from build123d import *

# Parameters (mm, degrees)
BOSS_EXTRUDE1_DEPTH = 6.35
SKETCH3_R           = 12.7
CUT_EXTRUDE1_DEPTH  = 3.175
SKETCH5_R           = 12.7
CUT_EXTRUDE2_DEPTH  = 3.175
SKETCH6_R           = 3.175
BOSS_EXTRUDE2_DEPTH = 25.4
FILLET1_R           = 2.54


with BuildPart() as part:
    # Sketch2 → Boss-Extrude1 (new body)
    with BuildSketch(Plane(origin=(0, 0, 0), x_dir=(1, 0, 0), z_dir=(0, 1, 0))):
        with BuildLine():
            ThreePointArc((0, -6.090706035), (29.21, 0), (0, 6.090706035))
            ThreePointArc((0, 6.090706035), (-29.21, 0), (0, -6.090706035))
        make_face()
    extrude(amount=BOSS_EXTRUDE1_DEPTH)

    # Sketch3 → Cut-Extrude1 (cut)
    with BuildSketch(Plane(origin=(0, 6.35, 0), x_dir=(1, 0, 0), z_dir=(0, 1, 0))):
        with Locations(Location((-13.959659088, 0, 0), (0, 0, 270))):
            Circle(SKETCH3_R)
    extrude(amount=-CUT_EXTRUDE1_DEPTH, mode=Mode.SUBTRACT)

    # Sketch5 → Cut-Extrude2 (cut)
    with BuildSketch(Plane(origin=(0, 6.35, 0), x_dir=(1, 0, 0), z_dir=(0, 1, 0))):
        with Locations(Location((14.045562682, 0, 0), (0, 0, 270))):
            Circle(SKETCH5_R)
    extrude(amount=-CUT_EXTRUDE2_DEPTH, mode=Mode.SUBTRACT)

    # Sketch6 → Boss-Extrude2 (add)
    with BuildSketch(Plane(origin=(0, 0, 0), x_dir=(-1, 0, 0), z_dir=(0, -1, 0))):
        with Locations(Location((0, 0, 0), (0, 0, 270))):
            Circle(SKETCH6_R)
    extrude(amount=BOSS_EXTRUDE2_DEPTH)

    # Fillet1
    fillet1_edges = [part.edges().sort_by_distance(p)[0] for p in [
        (0, 0, -3.175),
        (0, 3.175, -6.090706035),
        (0, 3.175, 6.090706035),
    ]]
    fillet(fillet1_edges, radius=FILLET1_R)


solid = part.part
For this review, take the finished solid that the model builds, in its own axes (mm). A direction names the side the tool comes from. Give positions to 0.01 mm unless a question says otherwise; leave off trailing zeros. Loops run counter-clockwise (first coordinate to the right, second up) from the corner with the lowest first, then second, coordinate; pieces in that order, holes last.
Item 1: Take a section at D-D, the plane x = -17. State the section outline as (y, z) points (3 decimals), and give its area (3 significant figures).
Item 2: Tool access review of faces 1 (the cylindrical face through (-29.2, 3.1, -0.5)), 2 (the cylindrical face through (26.637, 4.785, -1.653)): name each direction out of +Z, -Z, +X, -X, +Y, -Y from which nothing blocks a thin tool from reaching the whole face with its end or side.
Item 3: Take a section at C-C, the plane y = -8.5. State the section outline as (x, z) points (3 decimals).
Item 4: Take a section at A-A, the plane z = 0. State the section outline as (x, y) points (3 decimals).
Item 5: Take a section at B-B, the plane z = 10.5. State the section outline as (x, y) points (3 decimals).
Item 6: Insertion check: pin 1 (15 mm diameter, centred on x = 14.05, z = 0, fed in from +Y) (3 decimals); pin 2 (1.5 mm diameter, centred on y = -2.5, z = 0.5, fed in from +X); pin 3 (10 mm diameter, centred on x = 3.5, y = -19.5, fed in from -Z) (3 decimals). Each pin has a flat end and moves straight along its axis. Give the tip position at first contact, or say it passes through.
Item 7: For line 1 along X through (y, z) = (5, 0); line 2 along Y through (x, z) = (20.5, -12.5); line 3 along Y through (x, z) = (-15, 11.5) (3 decimals), list the stretches that pass through material, from the lowest coordinate up.
Item 8: Draft analysis for pull direction Z (two halves, no side actions). For faces 3 (the flat face through (-14, 3.175, 0)), 4 (the flat face through (0, -25.4, 0)), 5 (the cylindrical face through (1.93, -13.81, -2.52)), 6 (the flat face through (14, 3.175, 0)), state which applies: +Z half, -Z half, draft (parallel to the pull), parting line (faces both ways), or undercut.
Calculated:
1. outline: (0, -14.936) - (6.35, -14.936) - (6.35, -12.331) - (3.175, -12.331) - (3.175, 12.331) - (6.35, 12.331) - (6.35, 14.936) - (0, 14.936) - close
1. area: 111 mm2
2. face 1: +Y, -Y
2. face 2: +Y
3. outline: circle Ø6.35 at (0, 0)
4. outline: (-29.21, 0) - (-5.715, 0) arc R2.54 cw to (-3.175, -2.54) - (-3.175, -25.4) - (3.175, -25.4) - (3.175, -2.54) arc R2.54 cw to (5.715, 0) - (29.21, 0) - (29.21, 6.35) - (26.746, 6.35) - (26.746, 3.175) - (1.346, 3.175) - (1.346, 6.35) - (-1.26, 6.35) - (-1.26, 3.175) - (-26.66, 3.175) - (-26.66, 6.35) - (-29.21, 6.35) - close
5. outline: (-25.016, 0) - (-2.924, 0) - (-2.924, 6.35) - (-6.815, 6.35) - (-6.815, 3.175) - (-21.104, 3.175) - (-21.104, 6.35) - (-25.016, 6.35) - close; (2.924, 0) - (25.016, 0) - (25.016, 6.35) - (21.19, 6.35) - (21.19, 3.175) - (6.901, 3.175) - (6.901, 6.35) - (2.924, 6.35) - close
6. pin 1: stops at y = 3.175
6. pin 2: stops at x = 3.28
6. pin 3: stops at z = -3.175
7. line 1: x = -29.21 to -26.66, -1.26 to 1.35, 26.75 to 29.21
7. line 2: y = 0 to 6.35
7. line 3: y = 0 to 3.175
8. face 3: undercut
8. face 4: draft
8. face 5: parting line
8. face 6: undercut
